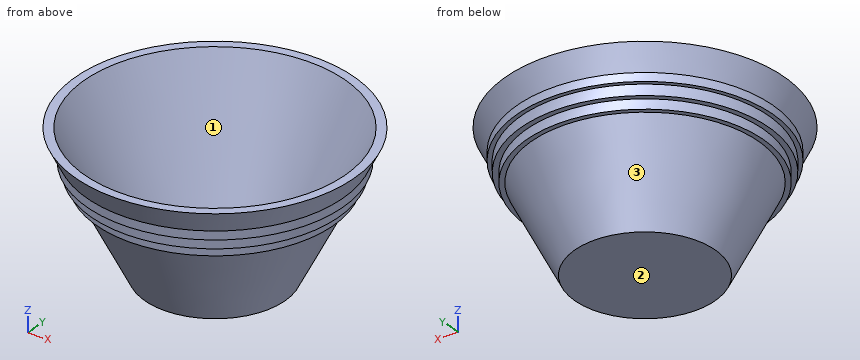
```python
from build123d import *


with BuildPart() as f1:
    # F0 (on Front) → F1 (revolve)
    with BuildSketch(Plane.XZ):
        Polygon((25.4, 0), (0, 0), (0, -3.0734), (27.299466, -3.0734), (44.208006, 30.743681), (46.09435, 34.516368), (48.180423, 38.688514), (49.815372, 41.958412), (54.236166, 50.8), (50.8, 50.8), align=None)
        Polygon((46.09435, 34.516368), (44.208006, 30.743681), (46.09435, 30.743681), align=None)
        Polygon((48.180423, 38.688514), (46.09435, 34.516368), (48.180423, 34.516368), align=None)
        Polygon((49.815372, 38.688514), (49.815372, 41.958412), (48.180423, 38.688514), align=None)
    revolve(axis=Axis((0, 0, 25.4), (0, 0, 1)))


solid = f1.part
```
Verification items for the finished model (mm, model axes). Face numbers are marked on the shaded views. Give positions to 0.01 mm unless a question says otherwise; leave off trailing zeros. Write each loop counter-clockwise with the first axis right and the second up, starting at its lowest first coordinate (ties: lowest second). Pieces come first, ordered by that corner, then holes. Notation, with made-up numbers: M -6,-24 L 20,-24 A9 cw 20,-15 Z; hole C 65,35 d1. An arc over 180 degrees is marked long. One line per question, with ' | ' between items.
1) Section check A-A on y = 0. Enter the section's corners in (x, z), plus the area to 3 significant figures.
Result:
outline: M -54.24,50.8 L -49.82,41.96 L -49.82,38.69 L -48.18,38.69 L -48.18,34.52 L -46.09,34.52 L -46.09,30.74 L -44.21,30.74 L -27.3,-3.07 L 27.3,-3.07 L 44.21,30.74 L 46.09,30.74 L 46.09,34.52 L 48.18,34.52 L 48.18,38.69 L 49.82,38.69 L 49.82,41.96 L 54.24,50.8 L 50.8,50.8 L 25.4,0 L -25.4,0 L -50.8,50.8 Z | area: 543 mm2
2) Section check C-C on z = 16. Enter the section's corners in (x, y).
Result:
outline: C 0,0 d73.67; hole C 0,0 d66.8
3) Gauge pin test, flat ends, axial feed: pin 1 Ø6 at (x, y) = (41.5, 17.5) entering from +Z; pin 2 Ø4 at (x, z) = (25.5, 7.5) entering from +Y; pin 3 Ø4 at (x, y) = (10.5, -12.5) entering from +Z. Record the tip position at first contact, or that the pin passes through.
Result:
pin 1: stops at z = 45.28 | pin 2: stops at y = 23.03 | pin 3: stops at z = 0
4) Mould release check, pull along Y, two halves, no side actions. Record for the marked faces 1, 2 and 3: released by +Y, released by -Y, zero draft, split by the parting line, or undercut.
Result:
face 1: undercut | face 2: zero draft | face 3: split by the parting line
5) Thickness scan on line 1 along Z through (x, y) = (-6, -8.5); line 2 along Y through (x, z) = (19, 1); line 3 along Y through (x, z) = (22, 23). Record the ranges inside material, lowest first. Write a range as [from, to].
Result:
line 1: z = [-3.07, 0] | line 2: y = [-22.35, -17.6], [17.6, 22.35] | line 3: y = [-33.81, -29.62], [29.62, 33.81]
